```python
from build123d import *

# Parameters (mm, degrees)
EXTRUDE_1_DEPTH = 20
EXTRUDE_4_DEPTH = 20
SKETCH_10_W     = 40
SKETCH_10_H     = 18
EXTRUDE_5_DEPTH = 20
SKETCH_11_R     = 7
SKETCH_11_R_2   = 6
EXTRUDE_6_DEPTH = 4
SKETCH_12_R     = 6
EXTRUDE_7_DEPTH = 4


with BuildPart() as part:
    # 草图2 → 凸台-拉伸1 (new body, symmetric)
    with BuildSketch(Plane(origin=(0, 0, 0), x_dir=(0, 0, -1), z_dir=(1, 0, 0))):
        Polygon((-10, 1), (10, 1), (10, -1), (-10, -1), (-12, -1), (-12, 1), align=None)
    extrude(amount=EXTRUDE_1_DEPTH, both=True)

    # 草图9 → 凸台-拉伸4 (add)
    with BuildSketch(Plane(origin=(0, 1, 0), x_dir=(1, 0, 0), z_dir=(0, 1, 0))):
        with BuildLine():
            Line((-40, -8), (40, -8))
            ThreePointArc((40, -8), (99.39696962, -32.60303038), (124, -92))
            Line((124, -92), (124, -108))
            Line((124, -108), (120, -108))
            Line((120, -108), (120, -92))
            ThreePointArc((120, -92), (96.568542495, -35.431457505), (40, -12))
            Line((40, -12), (-40, -12))
            ThreePointArc((-40, -12), (-96.568542495, -35.431457505), (-120, -92))
            Line((-120, -92), (-120, -108))
            Line((-120, -108), (-124, -108))
            Line((-124, -108), (-124, -92))
            ThreePointArc((-124, -92), (-99.39696962, -32.60303038), (-40, -8))
        make_face()
    extrude(amount=EXTRUDE_4_DEPTH)

    # 草图10 → 凸台-拉伸5 (add)
    with BuildSketch(Plane(origin=(0, 1, 0), x_dir=(1, 0, 0), z_dir=(0, 1, 0))):
        with Locations((0, 1)):
            Rectangle(SKETCH_10_W, SKETCH_10_H)
    extrude(amount=EXTRUDE_5_DEPTH)

    # 草图11 → 凸台-拉伸6 (add)
    with BuildSketch(Plane(origin=(0, 21, 0), x_dir=(1, 0, 0), z_dir=(0, 1, 0))):
        with Locations((0, -2.5)):
            Circle(SKETCH_11_R)
        with Locations((0, -2.5)):
            Circle(SKETCH_11_R_2, mode=Mode.SUBTRACT)
    extrude(amount=EXTRUDE_6_DEPTH)

    # 草图12 → 凸台-拉伸7 (add)
    with BuildSketch(Plane.XZ.offset(1)):
        with Locations((0, 2.5)):
            Circle(SKETCH_12_R)
    extrude(amount=EXTRUDE_7_DEPTH)


solid = part.part
```
Build history of the part. All positions in model axes, mm. A direction names the side the tool comes from. Give positions to 0.01 mm unless a question says otherwise; leave off trailing zeros. Loops run counter-clockwise (first coordinate to the right, second up) from the corner with the lowest first, then second, coordinate; pieces in that order, holes last.
1) Band-saw the part on C-C on y = 13.5. List the corners of the cut face in (x, z), then the cut area to 3 significant figures.
Values follow:
outline: (-124, 92) arc R84 ccw to (-40, 8) - (-20, 8) - (-20, -10) - (20, -10) - (20, 8) - (40, 8) arc R84 ccw to (124, 92) - (124, 108) - (120, 108) - (120, 92) arc R80 cw to (40, 12) - (-40, 12) arc R80 cw to (-120, 92) - (-120, 108) - (-124, 108) - close
area: 2,200 mm2
2) Drop flat-ended pins along their axis: P1, Ø14, axis at x = 0, z = 2.5, coming from the +Y side; P2, Ø5, axis at x = 5.5, z = 13, coming from the +Y side; P3, Ø10, axis at x = 98.5, y = 13, coming from the -Z side; P4, Ø4, axis at x = -84, y = 2.5, coming from the -Z side. Give the stop position or say it passes through.
Values follow:
P1: stops at y = 25
P2: stops at y = 21
P3: stops at z = 27.24
P4: stops at z = 19.25
3) 3-axis set-ups, long thin cutter, end or side, ignore diameter. For faces 1 (the face through (30, 11, 8)), 2 (the face through (-95, 1, 32)), 3 (the face through (-1.517, 22.972, 9.334)): which of +Z, -Z, +X, -X, +Y, -Y reach the whole face in a straight line?
Values follow:
face 1: -Z, +X, +Y, -Y
face 2: +Z, -Z, -X, -Y
face 3: +Y
4) Band-saw the part on A-A on z = 94.5. List the corners of the cut face in (x, y).
Values follow:
outline: (-124, 1) - (-120, 1) - (-120, 21) - (-124, 21) - close; (120, 1) - (124, 1) - (124, 21) - (120, 21) - close
5) Band-saw the part on D-D on z = 58. List the corners of the cut face in (x, y), then the cut area to 3 significant figures.
Values follow:
outline: (-116.81, 1) - (-112.42, 1) - (-112.42, 21) - (-116.81, 21) - close; (112.42, 1) - (116.81, 1) - (116.81, 21) - (112.42, 21) - close
area: 176 mm2
6) Band-saw the part on B-B on x = 0. List the corners of the cut face in (y, z).
Values follow:
outline: (-5, -3.5) - (-1, -3.5) - (-1, -10) - (21, -10) - (21, -4.5) - (25, -4.5) - (25, -3.5) - (21, -3.5) - (21, 8.5) - (25, 8.5) - (25, 9.5) - (21, 9.5) - (21, 12) - (-1, 12) - (-1, 8.5) - (-5, 8.5) - close
7) Probe line 1 along X through (y, z) = (23.25, 2.5); line 2 along Z through (x, y) = (0, 22.2); line 3 along X through (y, z) = (18.25, 102). List the from-to ranges inside material, lowest first.
Values follow:
line 1: x = -7 to -6, 6 to 7
line 2: z = -4.5 to -3.5, 8.5 to 9.5
line 3: x = -124 to -120, 120 to 124
8) Two-plate mould, pull along X, no slides. Class faces 4 (the face through (1, 10, 12)), 5 (the face through (98.74, 10.86, 31.954)), 6 (the face through (0, -1, -4)): released by +X, released by -X, zero draft, split by the parting line, or undercut.
Values follow:
face 4: undercut
face 5: released by +X
face 6: zero draft
